Geometry check sheet. Reference: the model listing, model coordinates, mm. Face numbers are marked on the shaded views. A direction names the side the tool comes from. Give positions to 0.01 mm unless a question says otherwise; leave off trailing zeros. Write each loop counter-clockwise with the first axis right and the second up, starting at its lowest first coordinate (ties: lowest second). Pieces come first, ordered by that corner, then holes. Notation, with made-up numbers: M -35,-37.5 L 8,-37.5 A30 ccw 8,-1.5 Z; hole C 82.25,18 d5. An arc over 180 degrees is marked long. One line per item, written item: value. Start each with the question number.
1. Cross-section at B-B on y = 25.25. Record the cut outline in (x, z) (3 decimals), then the cut area to 3 significant figures.
2. Tool access check on the marked faces 5 and 6. Record the directions out of +Z, -Z, +X, -X, +Y, -Y that give a thin tool (end or side, any length) a straight path to the whole face; none if there is none.
3. Scan lines: line 1 (Y direction, x = 45.15, z = 11.75) (3 decimals); line 2 (X direction, y = 28, z = 21.5); line 3 (Y direction, x = 36.5, z = 3.75). Record each from-to range of solid material in increasing order.
4. Cross-section at C-C on z = 11.5. Count the separate pieces of the cut face and the enclosed holes in it, then the cut area to 3 significant figures.
5. Cross-section at D-D on y = 4. Record the cut outline in (x, z), then the cut area to 3 significant figures.
6. Release check for a two-part mould opening along Y. For the marked faces 1, 2, 3 and 4 record: pulls with the +Y half, pulls with the -Y half, needs draft (parallel to the pull), parting line crosses it, or undercut.
7. Cross-section at A-A on x = -4.15. Record the cut outline in (y, z) (3 decimals).
from build123d import *

# Parameters (mm, degrees)
SKETCH1_W           = 57.6
SKETCH1_H           = 57.1
SKETCH1_R           = 1.125
SKETCH1_W_2         = 41
SKETCH1_H_2         = 40.5
BOSS_EXTRUDE1_DEPTH = 28
FILLET1_R           = 2.5


with BuildPart() as part:
    # Sketch1 → Boss-Extrude1 (new body)
    with BuildSketch(Plane.XY):
        with Locations((20.5, 20.25)):
            Rectangle(SKETCH1_W, SKETCH1_H)
        with Locations((-4.15, 25.25)):
            Circle(SKETCH1_R, mode=Mode.SUBTRACT)
        with Locations((-4.15, 30.25)):
            Circle(SKETCH1_R, mode=Mode.SUBTRACT)
        with Locations(Location((-4.15, 10.25, 0), (0, 0, 180))):
            Circle(SKETCH1_R, mode=Mode.SUBTRACT)
        with Locations(Location((-4.15, 15.25, 0), (0, 0, 180))):
            Circle(SKETCH1_R, mode=Mode.SUBTRACT)
        with Locations((45.15, 15.25)):
            Circle(SKETCH1_R, mode=Mode.SUBTRACT)
        with Locations((45.15, 10.25)):
            Circle(SKETCH1_R, mode=Mode.SUBTRACT)
        with Locations(Location((45.15, 30.25, 0), (0, 0, 180))):
            Circle(SKETCH1_R, mode=Mode.SUBTRACT)
        with Locations(Location((45.15, 25.25, 0), (0, 0, 180))):
            Circle(SKETCH1_R, mode=Mode.SUBTRACT)
        with Locations((20.5, 20.25)):
            Rectangle(SKETCH1_W_2, SKETCH1_H_2, mode=Mode.SUBTRACT)
    extrude(amount=BOSS_EXTRUDE1_DEPTH)

    # Fillet1
    fillet1_edges = [part.edges().sort_by_distance(p)[0] for p in [
        (-8.3, 48.8, 14),
        (49.3, 48.8, 14),
        (49.3, -8.3, 14),
        (-8.3, -8.3, 14),
    ]]
    fillet(fillet1_edges, radius=FILLET1_R)


solid = part.part
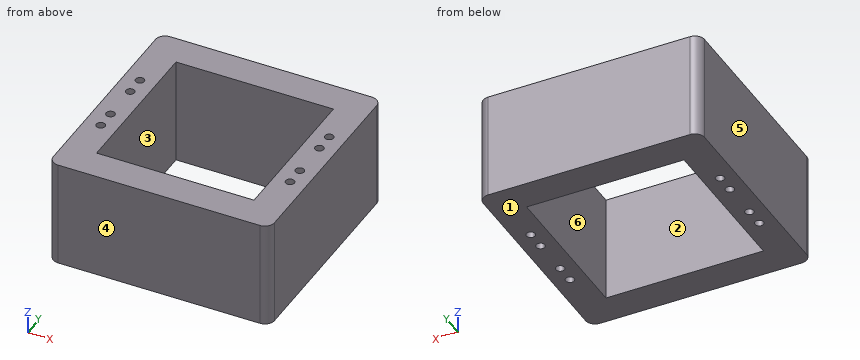
Report:
1. outline: M -8.3,0 L -5.275,0 L -5.275,28 L -8.3,28 Z; M -3.025,0 L 0,0 L 0,28 L -3.025,28 Z; M 41,0 L 44.025,0 L 44.025,28 L 41,28 Z; M 46.275,0 L 49.3,0 L 49.3,28 L 46.275,28 Z
1. area: 339 mm^2
2. face 5: +Z, -Z, -X, +Y, -Y
2. face 6: +Z, -Z
3. line 1: y = -8.3 to 9.125, 11.375 to 14.125, 16.375 to 24.125, 26.375 to 29.125, 31.375 to 48.8
3. line 2: x = -8.3 to 0, 41 to 49.3
3. line 3: y = -8.3 to 0, 40.5 to 48.8
4. separate pieces: 1
4. enclosed holes: 9
4. area: 1,590 mm^2
5. outline: M -8.3,0 L 0,0 L 0,28 L -8.3,28 Z; M 41,0 L 49.3,0 L 49.3,28 L 41,28 Z
5. area: 465 mm^2
6. face 1: needs draft
6. face 2: undercut
6. face 3: undercut
6. face 4: pulls with the -Y half
7. outline: M -8.3,0 L 9.125,0 L 9.125,28 L -8.3,28 Z; M 11.375,0 L 14.125,0 L 14.125,28 L 11.375,28 Z; M 16.375,0 L 24.125,0 L 24.125,28 L 16.375,28 Z; M 26.375,0 L 29.125,0 L 29.125,28 L 26.375,28 Z; M 31.375,0 L 48.8,0 L 48.8,28 L 31.375,28 Z
